Geometry: final body of the model. Coordinates: model frame, mm. Face numbers are marked on the shaded views. A direction names the side the tool comes from. Round coordinates to 2 decimals unless told otherwise and drop trailing zeros. Order: outer loops, then holes, each group sorted by start corner. A loop starts at its lowest first (then second) coordinate and runs counter-clockwise, first axis right, second up. Notation, with made-up numbers: M 75.25,89 L 102.25,89 A15 cw 102.25,118 Z; hole C 86.5,4 d5. An arc over 180 degrees is marked long. Return JSON: item names as keys, results as strings. Group by question number.
Q1. Access query for the marked faces 1 and 2. Directions: +Z, -Z, +X, -X, +Y, -Y. A direction counts if a zero-diameter tool reaches every point of the face in a straight line with its end or side. Return the directions, or none.
Q2. Contact query for flat-ended pins moving along their axis: pin 1 (17.5 mm diameter, centred on y = -4, z = 82.5, fed in from +X); pin 2 (12 mm diameter, centred on x = 13, z = 71, fed in from -Y); pin 3 (3 mm diameter, centred on x = 65.5, z = 63.5, fed in from +Y); pin 4 (1.5 mm diameter, centred on x = 29.5, y = 23, fed in from +Z). Output: stop coordinate, or through.
Q3. Cut plane B-B on z = 84. Output: boundary loops of the cut face in (x, y).
Q4. Cut plane A-A on x = 67. Output: boundary loops of the cut face in (y, z).
Q5. Ray query, probe 1 along X at (y, z) = (4.5, 67.5); probe 2 along X at (y, z) = (-31, 71); probe 3 along Z at (x, y) = (134, -16). Return the intervals inside material, ascending.
Q6. Cut plane D-D on z = 72.5. Count the separate pieces of the cut face and the enclosed holes in it, and give its area (3 significant figures).
Q7. Cut plane C-C on x = 131. Output: boundary loops of the cut face in (y, z).
```python
from build123d import *

# Parameters (mm, degrees)
EXTRUDE_1_DEPTH      = 30
SKETCH_2_R           = 44.45
CUT_EXTRUDE_1_DEPTH  = 4
SKETCH_3_R           = 25.5
SKETCH_3_R_2         = 2.25
CUT_EXTRUDE_2_DEPTH  = 188.619295383
CUT_EXTRUDE_3_DEPTH  = 189.215302247
SKETCH_5_R           = 1.65
CUT_EXTRUDE_4_DEPTH  = 189.215302247
EXTRUDE_START        = -30
EXTRUDE_2_DEPTH      = 30
CUT_EXTRUDE_5_DEPTH  = 198.040604952
CUT_EXTRUDE_7_DEPTH  = 233.432785983
CUT_EXTRUDE_8_DEPTH  = 233.432785983
CUT_EXTRUDE_9_DEPTH  = 233.432785983
FILLET_1_R           = 5
CUT_EXTRUDE_10_DEPTH = 233.432785983
EXTRUDE_START_2      = -5
EXTRUDE_3_DEPTH      = 5
EXTRUDE_4_DEPTH      = 5
SKETCH_14_R          = 4.25
CUT_EXTRUDE_11_DEPTH = 189.364728478
SKETCH_16_W          = 43
SKETCH_16_H          = 30
CUT_EXTRUDE_12_DEPTH = 233.432785983
EXTRUDE_7_REACH      = 188.592
SKETCH_18_W          = 210
SKETCH_18_H          = 5
EXTRUDE_8_DEPTH      = 210
EXTRUDE_9_DEPTH      = 5
EXTRUDE_10_DEPTH     = 5
SKETCH_22_R          = 4.25
CUT_EXTRUDE_13_DEPTH = 187.984035343
FILLET_2_R           = 5
SKETCH_23_W          = 158.512158041
SKETCH_23_H          = 103.317713915
CUT_EXTRUDE_14_DEPTH = 234.418610938


with BuildPart() as part:
    # 草图1 → 凸台-拉伸1 (new body)
    with BuildSketch(Plane(origin=(0, 0, 0), x_dir=(1, 0, 0), z_dir=(0, 1, 0))):
        with BuildLine():
            Line((170, 31.93), (170, -31.93))
            ThreePointArc((170, -31.93), (167.781993847, -38.210172909), (162.111885646, -41.704453387))
            Line((162.111885646, -41.704453387), (15.839142344, -73.308400404))
            ThreePointArc((15.839142344, -73.308400404), (-75, 0), (15.839142344, 73.308400404))
            Line((15.839142344, 73.308400404), (162.111885646, 41.704453387))
            ThreePointArc((162.111885646, 41.704453387), (167.781993847, 38.210172909), (170, 31.93))
        make_face()
    extrude(amount=EXTRUDE_1_DEPTH)

    # 草图2 → 切除-拉伸1 (cut)
    with BuildSketch(Plane(origin=(0, 30, 0), x_dir=(1, 0, 0), z_dir=(0, 1, 0))):
        with Locations(Location((0, 0, 0), (0, 0, 270))):
            Circle(SKETCH_2_R)
    extrude(amount=-CUT_EXTRUDE_1_DEPTH, mode=Mode.SUBTRACT)

    # 草图3 → 切除-拉伸2 (cut, through all)
    with BuildSketch(Plane(origin=(0, 26, 0), x_dir=(1, 0, 0), z_dir=(0, 1, 0))):
        with Locations(Location((0, 0, 0), (0, 0, 270))):
            Circle(SKETCH_3_R)
        with Locations(Location((0, 41, 0), (0, 0, 270))):
            Circle(SKETCH_3_R_2)
        with Locations(Location((28.991378029, 28.991378029, 0), (0, 0, 270))):
            Circle(SKETCH_3_R_2)
        with Locations(Location((41, 0, 0), (0, 0, 270))):
            Circle(SKETCH_3_R_2)
        with Locations(Location((28.991378029, -28.991378029, 0), (0, 0, 270))):
            Circle(SKETCH_3_R_2)
        with Locations(Location((0, -41, 0), (0, 0, 270))):
            Circle(SKETCH_3_R_2)
        with Locations(Location((-28.991378029, -28.991378029, 0), (0, 0, 270))):
            Circle(SKETCH_3_R_2)
        with Locations(Location((-41, 0, 0), (0, 0, 270))):
            Circle(SKETCH_3_R_2)
        with Locations(Location((-28.991378029, 28.991378029, 0), (0, 0, 270))):
            Circle(SKETCH_3_R_2)
    extrude(amount=-CUT_EXTRUDE_2_DEPTH, mode=Mode.SUBTRACT)

    # 草图4 → 切除-拉伸3 (cut, through all)
    with BuildSketch(Plane(origin=(0, 30, 0), x_dir=(1, 0, 0), z_dir=(0, 1, 0))):
        with BuildLine():
            Line((124, 18.5), (134, 18.5))
            ThreePointArc((134, 18.5), (152.5, 0), (134, -18.5))
            Line((134, -18.5), (124, -18.5))
            ThreePointArc((124, -18.5), (105.5, 0), (124, 18.5))
        make_face()
    extrude(amount=-CUT_EXTRUDE_3_DEPTH, mode=Mode.SUBTRACT)

    # 草图5 → 切除-拉伸4 (cut, through all)
    with BuildSketch(Plane(origin=(0, 30, 0), x_dir=(1, 0, 0), z_dir=(0, 1, 0))):
        with Locations(Location((116.75, 25.5, 0), (0, 0, 270))):
            Circle(SKETCH_5_R)
        with Locations(Location((141.25, 25.5, 0), (0, 0, 270))):
            Circle(SKETCH_5_R)
        with Locations(Location((141.25, -25.5, 0), (0, 0, 270))):
            Circle(SKETCH_5_R)
        with Locations(Location((116.75, -25.5, 0), (0, 0, 270))):
            Circle(SKETCH_5_R)
    extrude(amount=-CUT_EXTRUDE_4_DEPTH, mode=Mode.SUBTRACT)

    # 草图6 → 凸台-拉伸2 (add)
    with BuildSketch(Plane(origin=(0, 30, 0), x_dir=(1, 0, 0), z_dir=(0, 1, 0)).offset(EXTRUDE_START)):
        with BuildLine():
            Line((158, 95), (-52, 95))
            Line((-52, 95), (-52, 54.046276467))
            ThreePointArc((-52, 54.046276467), (-20.48558667, 72.148047366), (15.839142344, 73.308400404))
            Line((15.839142344, 73.308400404), (158, 42.592874655))
            Line((158, 42.592874655), (158, 95))
        make_face()
        with BuildLine():
            ThreePointArc((15.839142344, -73.308400404), (-20.48558667, -72.148047366), (-52, -54.046276467))
            Line((-52, -54.046276467), (-52, -95))
            Line((-52, -95), (158, -95))
            Line((158, -95), (158, -42.592874655))
            Line((158, -42.592874655), (15.839142344, -73.308400404))
        make_face()
    extrude(amount=EXTRUDE_2_DEPTH)

    # 草图7 → 切除-拉伸5 (cut, through all)
    with BuildSketch(Plane(origin=(0, 30, 0), x_dir=(1, 0, 0), z_dir=(0, 1, 0))):
        with BuildLine():
            Line((-52, 54.046276467), (-52, -54.046276467))
            ThreePointArc((-52, -54.046276467), (-75, 0), (-52, 54.046276467))
        make_face()
        with BuildLine():
            Line((158, 42.592874655), (158, -42.592874655))
            Line((158, -42.592874655), (162.111885646, -41.704453387))
            ThreePointArc((162.111885646, -41.704453387), (167.781993847, -38.210172909), (170, -31.93))
            Line((170, -31.93), (170, 31.93))
            ThreePointArc((170, 31.93), (167.781993847, 38.210172909), (162.111885646, 41.704453387))
            Line((162.111885646, 41.704453387), (158, 42.592874655))
        make_face()
    extrude(amount=-CUT_EXTRUDE_5_DEPTH, mode=Mode.SUBTRACT)

    # 草图9 → 切除-拉伸7 (cut, through all)
    with BuildSketch(Plane.ZY.offset(52)):
        Polygon((-95, 20), (-60, 10.621778265), (-60, 30), (-95, 30), align=None)
    extrude(amount=-CUT_EXTRUDE_7_DEPTH, mode=Mode.SUBTRACT)

    # 草图10 → 切除-拉伸8 (cut, through all)
    with BuildSketch(Plane.ZY.offset(52)):
        Polygon((-95, 12.753066737), (-52, 1.231251463), (-52, 0), (-95, 0), align=None)
    extrude(amount=-CUT_EXTRUDE_8_DEPTH, mode=Mode.SUBTRACT)

    # 草图8 → 切除-拉伸9 (cut, through all)
    with BuildSketch(Plane.ZY.offset(52)):
        Polygon((0, 0), (52, 0), (52, 17.3), (-52, 17.3), (-52, 0), align=None)
    extrude(amount=-CUT_EXTRUDE_9_DEPTH, mode=Mode.SUBTRACT)

    # 圆角1
    fillet_1_edges = [part.edges().sort_by_distance(p)[0] for p in [
        (53, 10.621778265, -60),
    ]]
    fillet(fillet_1_edges, radius=FILLET_1_R)

    # 草图11 → 切除-拉伸10 (cut, through all)
    with BuildSketch(Plane.ZY.offset(52)):
        Polygon((-95, 12.753066737), (-93.188266684, 19.514547521), (-95, 20), align=None)
    extrude(amount=-CUT_EXTRUDE_10_DEPTH, mode=Mode.SUBTRACT)

    # 草图12 → 凸台-拉伸3 (add)
    with BuildSketch(Plane.ZY.offset(52).offset(EXTRUDE_START_2)):
        with BuildLine():
            Line((-93.188266684, 19.514547521), (-60, 30))
            Line((-60, 30), (-60, 17.137905129))
            ThreePointArc((-60, 17.137905129), (-61.956192855, 13.171138428), (-66.294095226, 12.308275998))
            Line((-66.294095226, 12.308275998), (-93.188266684, 19.514547521))
        make_face()
    extrude(amount=EXTRUDE_3_DEPTH)

    # 草图13 → 凸台-拉伸4 (add)
    with BuildSketch(Plane(origin=(158, 0, 0), x_dir=(0, 0, -1), z_dir=(1, 0, 0))):
        with BuildLine():
            Line((66.294095226, 12.308275998), (93.188266684, 19.514547521))
            Line((93.188266684, 19.514547521), (60, 30))
            Line((60, 30), (60, 17.137905129))
            ThreePointArc((60, 17.137905129), (61.956192855, 13.171138428), (66.294095226, 12.308275998))
        make_face()
    extrude(amount=-EXTRUDE_4_DEPTH)

    # 草图14 → 切除-拉伸11 (cut, through all)
    with BuildSketch(Plane(origin=(0, -5.089745962, -1.36379332), x_dir=(1, 0, 0), z_dir=(0, 0.9659258262890681, 0.2588190451025214))):
        with Locations(Location((-27, 82.063690052, 0), (0, 0, 270))):
            Circle(SKETCH_14_R)
        with Locations(Location((23, 82.063690052, 0), (0, 0, 270))):
            Circle(SKETCH_14_R)
        with Locations(Location((83, 82.063690052, 0), (0, 0, 270))):
            Circle(SKETCH_14_R)
        with Locations(Location((133, 82.063690052, 0), (0, 0, 270))):
            Circle(SKETCH_14_R)
    extrude(amount=-CUT_EXTRUDE_11_DEPTH, mode=Mode.SUBTRACT)

    # 草图16 → 切除-拉伸12 (cut, through all)
    with BuildSketch(Plane.ZY.offset(52)):
        with Locations((73.5, 15)):
            Rectangle(SKETCH_16_W, SKETCH_16_H)
    extrude(amount=-CUT_EXTRUDE_12_DEPTH, mode=Mode.SUBTRACT)

    # 凸台-拉伸7: up to this plane
    extrude_7_end = Plane(origin=(0, -11.851226746, -3.175526636), z_dir=(0, -0.9659258262890681, -0.25881904510252146))
    # 草图18 → 凸台-拉伸7 (add, up to the surface)
    with BuildSketch(Plane(origin=(0, 30, 0), x_dir=(1, 0, 0), z_dir=(0, 1, 0)), mode=Mode.PRIVATE) as extrude_7_sk1:
        with Locations((53, -54.5)):
            Rectangle(SKETCH_18_W, SKETCH_18_H)
    extrude_7_tool1 = split(extrude(extrude_7_sk1.sketch, amount=-EXTRUDE_7_REACH, mode=Mode.PRIVATE), bisect_by=extrude_7_end, keep=Keep.BOTH, mode=Mode.PRIVATE)
    add(extrude_7_tool1.solids().sort_by_distance((53, 30, 54.5))[0])

    # 草图19 → 凸台-拉伸8 (add)
    with BuildSketch(Plane.ZY.offset(52)):
        Polygon((57, -27.975210512), (90.188266684, -36.867979769), (92, -30.106498985), (57, -20.72827725), align=None)
    extrude(amount=-EXTRUDE_8_DEPTH)

    # 草图20 → 凸台-拉伸9 (add)
    with BuildSketch(Plane.ZY.offset(52)):
        Polygon((92, -30.106498985), (57, -20.72827725), (57, 30), align=None)
    extrude(amount=-EXTRUDE_9_DEPTH)

    # 草图21 → 凸台-拉伸10 (add)
    with BuildSketch(Plane(origin=(158, 0, 0), x_dir=(0, 0, -1), z_dir=(1, 0, 0))):
        Polygon((-57, 30), (-92, -30.106498985), (-57, -20.72827725), align=None)
    extrude(amount=-EXTRUDE_10_DEPTH)

    # 草图22 → 切除-拉伸13 (cut, through all)
    with BuildSketch(Plane(origin=(0, -5.089745962, -1.36379332), x_dir=(1, 0, 0), z_dir=(0, 0.9659258262890686, 0.25881904510251946))):
        with Locations(Location((-27, -77.936309948, 0), (0, 0, 270))):
            Circle(SKETCH_22_R)
        with Locations(Location((23, -69.936309948, 0), (0, 0, 270))):
            Circle(SKETCH_22_R)
        with Locations(Location((83, -69.936309948, 0), (0, 0, 270))):
            Circle(SKETCH_22_R)
        with Locations(Location((133, -77.936309948, 0), (0, 0, 270))):
            Circle(SKETCH_22_R)
    extrude(amount=-CUT_EXTRUDE_13_DEPTH, mode=Mode.SUBTRACT)

    # 圆角2
    fillet_2_edges = [part.edges().sort_by_distance(p)[0] for p in [
        (53, -20.72827725, 57),
    ]]
    fillet(fillet_2_edges, radius=FILLET_2_R)

    # 草图23 → 切除-拉伸14 (cut, through all)
    with BuildSketch(Plane.ZY.offset(52)):
        with Locations((-27.256079021, 5.306767281)):
            Rectangle(SKETCH_23_W, SKETCH_23_H)
    extrude(amount=-CUT_EXTRUDE_14_DEPTH, mode=Mode.SUBTRACT)


solid = part.part
```
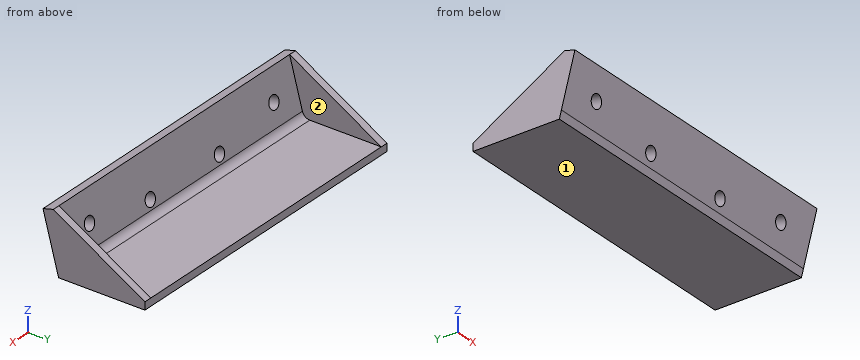
Result sheet:
{
 "1": {"face 1": "-Z, +X, -X, +Y, -Y", "face 2": "+Z, +Y"},
 "2": {"pin 1": "stops at x = 158", "pin 2": "stops at y = -33.33", "pin 3": "stops at y = -22.07", "pin 4": "stops at z = 57"},
 "3": {"outline": "M -52,-35.21 L 158,-35.21 L 158,-16.37 L 153,-16.37 L 153,-27.96 L -47,-27.96 L -47,-16.37 L -52,-16.37 Z"},
 "4": {"outline": "M -36.87,90.19 L -26.64,52 L 30,52 L 30,57 L -16.89,57 A5 cw -21.72,60.71 L -30.11,92 Z"},
 "5": {"probe 1": "x = -52 to -47, 153 to 158", "probe 2": "x = -52 to -31.04, -22.96 to 128.96, 137.04 to 158", "probe 3": "z = 52 to 57"},
 "6": {"separate pieces": "3", "enclosed holes": "0", "area": "1,680 mm²"},
 "7": {"outline": "M -36.87,90.19 L -32.99,75.73 L -26.23,77.54 L -30.11,92 Z; M -31.05,68.48 L -26.64,52 L 30,52 L 30,57 L -16.89,57 A5 cw -21.72,60.71 L -24.29,70.29 Z"}
}
